```python
from build123d import *

# Parameters (mm, degrees)
IZIM1_W                        = 65
IZIM1_H                        = 65
Y_KSEKLIK_EKSTR_ZYON1_DEPTH    = 6
IZIM2_R                        = 30.2
Y_KSEKLIK_EKSTR_ZYON2_DEPTH    = 53.5
IZIM3_W                        = 36
IZIM3_H                        = 6.950463922
Y_KSEKLIK_EKSTR_ZYON3_DEPTH    = 35
IZIM5_R                        = 1.5
KES_EKSTR_ZYON2_DEPTH          = 10
Y_KSEKLIK_EKSTR_ZYON7_START    = 10
IZIM31_R                       = 1.5
Y_KSEKLIK_EKSTR_ZYON7_DEPTH    = 10
M3_SFHCS_IN_HAV_A5_D           = 3.2
M3_SFHCS_IN_HAV_A5_DEPTH       = 10
M3_SFHCS_IN_HAV_A5_CSINK_D     = 6.72
M3_SFHCS_IN_HAV_A5_CSINK_ANGLE = 90
M3_SFHCS_IN_HAV_A5_TIP         = 0.96137699
Y_KSEKLIK_EKSTR_ZYON8_DEPTH    = 19
RADYUS1_R                      = 4
IZIM35_R                       = 29
KES_EKSTR_ZYON3_DEPTH          = 0.3
IZIM36_R                       = 15.75
Y_KSEKLIK_EKSTR_ZYON9_DEPTH    = 8
IZIM37_R                       = 10.75
KES_EKSTR_ZYON4_DEPTH          = 1
IZIM38_R                       = 4.75
Y_KSEKLIK_EKSTR_ZYON10_DEPTH   = 22
IZIM39_R                       = 2.5
KES_EKSTR_ZYON5_DEPTH          = 10
RADYUS2_R                      = 3


with BuildPart() as part:
    # Çizim1 → Yükseklik-Ekstrüzyon1 (new body)
    with BuildSketch(Plane.XY):
        Rectangle(IZIM1_W, IZIM1_H)
    extrude(amount=Y_KSEKLIK_EKSTR_ZYON1_DEPTH)

    # Çizim2 → Yükseklik-Ekstrüzyon2 (add)
    with BuildSketch(Plane(origin=(0, 0, 0), x_dir=(-1, 0, 0), z_dir=(0, 0, -1))):
        Circle(IZIM2_R)
    extrude(amount=Y_KSEKLIK_EKSTR_ZYON2_DEPTH)

    # Çizim3 → Yükseklik-Ekstrüzyon3 (add)
    with BuildSketch(Plane(origin=(0, 0, -53.5), x_dir=(-1, 0, 0), z_dir=(0, 0, -1))):
        with Locations((0, -27.724768039)):
            Rectangle(IZIM3_W, IZIM3_H)
    extrude(amount=-Y_KSEKLIK_EKSTR_ZYON3_DEPTH)

    # Çizim5 → Kes-Ekstrüzyon2 (cut)
    with BuildSketch(Plane(origin=(0, 0, -53.5), x_dir=(-1, 0, 0), z_dir=(0, 0, -1))):
        with Locations((0, 25.2)):
            Circle(IZIM5_R)
        with Locations((-17.819090886, -17.819090886)):
            Circle(IZIM5_R)
        with Locations((17.819090886, -17.819090886)):
            Circle(IZIM5_R)
    extrude(amount=-KES_EKSTR_ZYON2_DEPTH, mode=Mode.SUBTRACT)

    # Çizim31 → Yükseklik-Ekstrüzyon7 (add)
    with BuildSketch(Plane(origin=(0, 0, -43.5), x_dir=(-1, 0, 0), z_dir=(0, 0, -1)).offset(Y_KSEKLIK_EKSTR_ZYON7_START)):
        with Locations((0, 25.2)):
            Circle(IZIM31_R)
        with Locations((17.819090886, -17.819090886)):
            Circle(IZIM31_R)
        with Locations((-17.819090886, -17.819090886)):
            Circle(IZIM31_R)
    extrude(amount=-Y_KSEKLIK_EKSTR_ZYON7_DEPTH)

    # M3 SFHCS İçin Havşa5
    with Locations(Plane(origin=(0, 0, -53.5), x_dir=(-1, 0, 0), z_dir=(0, 0, -1))):
        with Locations((0, 25.2), (-17.819090886, -17.819090886), (17.819090886, -17.819090886)):
            CounterSinkHole(M3_SFHCS_IN_HAV_A5_D / 2, M3_SFHCS_IN_HAV_A5_CSINK_D / 2, depth=M3_SFHCS_IN_HAV_A5_DEPTH, counter_sink_angle=M3_SFHCS_IN_HAV_A5_CSINK_ANGLE)
            with Locations((0, 0, -(M3_SFHCS_IN_HAV_A5_DEPTH + M3_SFHCS_IN_HAV_A5_TIP / 2))):  # 118° drill point
                Cone(0, M3_SFHCS_IN_HAV_A5_D / 2, M3_SFHCS_IN_HAV_A5_TIP, mode=Mode.SUBTRACT)

    # Çizim34 → Yükseklik-Ekstrüzyon8 (add)
    with BuildSketch(Plane.XZ.offset(31.2)):
        Polygon((-8.660254038, -36), (-4.330127019, -43.5), (4.330127019, -43.5), (8.660254038, -36), (4.330127019, -28.5), (-4.330127019, -28.5), align=None)
    extrude(amount=Y_KSEKLIK_EKSTR_ZYON8_DEPTH)

    # Radyus1
    radyus1_edges = [part.edges().sort_by_distance(p)[0] for p in [
        (-6.495190528, -50.2, -32.25),
        (-6.495190528, -50.2, -39.75),
        (0, -50.2, -43.5),
        (6.495190528, -50.2, -39.75),
        (6.495190528, -50.2, -32.25),
        (0, -50.2, -28.5),
    ]]
    fillet(radyus1_edges, radius=RADYUS1_R)

    # Çizim35 → Kes-Ekstrüzyon3 (cut)
    with BuildSketch(Plane.XY.offset(6)):
        Circle(IZIM35_R)
    extrude(amount=-KES_EKSTR_ZYON3_DEPTH, mode=Mode.SUBTRACT)

    # Çizim36 → Yükseklik-Ekstrüzyon9 (add)
    with BuildSketch(Plane.XY.offset(5.7)):
        Circle(IZIM36_R)
    extrude(amount=Y_KSEKLIK_EKSTR_ZYON9_DEPTH)

    # Çizim37 → Kes-Ekstrüzyon4 (cut)
    with BuildSketch(Plane.XY.offset(13.7)):
        Circle(IZIM37_R)
    extrude(amount=-KES_EKSTR_ZYON4_DEPTH, mode=Mode.SUBTRACT)

    # Çizim38 → Yükseklik-Ekstrüzyon10 (add)
    with BuildSketch(Plane.XY.offset(12.7)):
        Circle(IZIM38_R)
    extrude(amount=Y_KSEKLIK_EKSTR_ZYON10_DEPTH)

    # Çizim39 → Kes-Ekstrüzyon5 (cut)
    with BuildSketch(Plane.XY.offset(6)):
        with Locations((26.5, -26.5)):
            Circle(IZIM39_R)
        with Locations((-26.5, -26.5)):
            Circle(IZIM39_R)
        with Locations((-26.5, 26.5)):
            Circle(IZIM39_R)
        with Locations((26.5, 26.5)):
            Circle(IZIM39_R)
    extrude(amount=-KES_EKSTR_ZYON5_DEPTH, mode=Mode.SUBTRACT)

    # Radyus2
    radyus2_edges = [part.edges().sort_by_distance(p)[0] for p in [
        (-32.5, 32.5, 3),
        (32.5, 32.5, 3),
        (32.5, -32.5, 3),
        (-32.5, -32.5, 3),
    ]]
    fillet(radyus2_edges, radius=RADYUS2_R)


solid = part.part
```
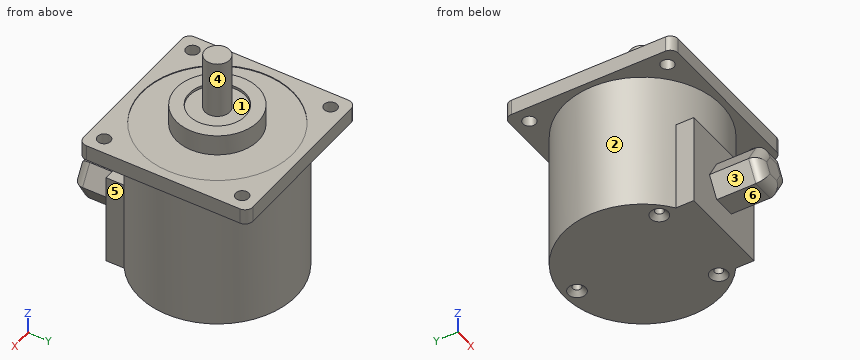
Model file for the job. Use its own axes, mm. Face numbers are marked on the shaded views. A direction names the side the tool comes from. Coordinates: 2 decimals unless noted, no trailing zeros. Order: outer loops, then holes, each group sorted by start corner. A loop starts at its lowest first (then second) coordinate and runs counter-clockwise, first axis right, second up. Notation, with made-up numbers: (56, 40.25) -> (96, 40.25) arc R4 cw to (96, 46.25) -> close; hole circle Ø2 at (-36.5, 8.5). An arc over 180 degrees is marked (long way). Answer as a JSON object with one key per item and string values. Group by question number.
1) Cut at A-A, the plane y = 0. Write the cut outline in (x, z).
2) Which spindle directions (+Z, -Z, +X, -X, +Y, -Y) get a long thin tool onto all of the face, cutting with end or side? Do the marked faces 4, 5 and 6. Say none if no direction does.
3) Cut at C-C, the plane z = -5. Write the cut outline in (x, y).
4) Cut at D-D, the plane x = -12. Write the cut outline in (y, z), then the cut area to 3 significant figures.
5) Pull direction Y, two halves, no side cores. Call the marked faces 1, 2 and 3: +Y half, -Y half, draft (parallel to the pull), parting line (faces both ways), or undercut.
6) Drill centre lines: L1, parallel to Y at x = 26.5, z = 2.35; L2, parallel to X at y = -17, z = -46; L3, parallel to Y at x = 0, z = -48. Where is each one in solid material? Low to high.
7) Cut at B-B, the plane x = -26.5. Write the cut outline in (y, z), then the cut area to 3 significant figures.
8) Flat gauge pins, fed straight in: pin 1 (9.5 mm diameter, centred on x = -1, y = -40.5, fed in from -Z); pin 2 (8 mm diameter, centred on x = -26.5, y = 26.5, fed in from -Z); pin 3 (3 mm diameter, centred on x = 11.5, z = 3, fed in from -Y); pin 4 (3 mm diameter, centred on x = 26.5, y = -26.5, fed in from +Z). Where does each tip first touch, or does it go through?
Check values:
{
 "1": {"outline": "(-32.5, 0) -> (-30.2, 0) -> (-30.2, -53.5) -> (30.2, -53.5) -> (30.2, 0) -> (32.5, 0) -> (32.5, 6) -> (29, 6) -> (29, 5.7) -> (15.75, 5.7) -> (15.75, 13.7) -> (10.75, 13.7) -> (10.75, 12.7) -> (4.75, 12.7) -> (4.75, 34.7) -> (-4.75, 34.7) -> (-4.75, 12.7) -> (-10.75, 12.7) -> (-10.75, 13.7) -> (-15.75, 13.7) -> (-15.75, 5.7) -> (-29, 5.7) -> (-29, 6) -> (-32.5, 6) -> close"},
 "2": {"face 4": "+Z", "face 5": "-Z, +X, -Y", "face 6": "-Z, +X, -X, -Y"},
 "3": {"outline": "circle Ø60.4 at (0, 0)"},
 "4": {"outline": "(-32.5, 0) -> (-27.71, 0) -> (-27.71, -18.5) -> (-31.2, -18.5) -> (-31.2, -53.5) -> (27.71, -53.5) -> (27.71, 0) -> (32.5, 0) -> (32.5, 6) -> (26.4, 6) -> (26.4, 5.7) -> (10.2, 5.7) -> (10.2, 13.7) -> (-10.2, 13.7) -> (-10.2, 5.7) -> (-26.4, 5.7) -> (-26.4, 6) -> (-32.5, 6) -> close", "area": "3,620 mm²"},
 "5": {"face 1": "undercut", "face 2": "parting line", "face 3": "draft"},
 "6": {"L1": "y = -32.5 to -29, -24 to 24, 29 to 32.5", "L2": "x = -24.96 to -19.19, -16.44 to 16.44, 19.19 to 24.96", "L3": "y = -31.2 to 23.6, 26.8 to 30.2"},
 "7": {"outline": "(-32.5, 0) -> (-29, 0) -> (-29, 6) -> (-32.5, 6) -> close; (-24, 0) -> (-14.48, 0) -> (-14.48, -53.5) -> (14.48, -53.5) -> (14.48, 0) -> (24, 0) -> (24, 6) -> (11.78, 6) -> (11.78, 5.7) -> (-11.78, 5.7) -> (-11.78, 6) -> (-24, 6) -> close; (29, 0) -> (32.5, 0) -> (32.5, 6) -> (29, 6) -> close", "area": "1,870 mm²"},
 "8": {"pin 1": "stops at z = -43.5", "pin 2": "stops at z = 0", "pin 3": "stops at y = -32.5", "pin 4": "passes through"}
}
